Answer from the drawing. Dimensions are ordinates in mm from the lowest x, y and z of the part. Round coordinates to 2 decimals unless told otherwise and drop trailing zeros. Loops run counter-clockwise (first coordinate to the right, second up) from the corner with the lowest first, then second, coordinate; pieces in that order, holes last. Notation, with made-up numbers: (29, -7.5) - (38, -7.5) arc R9 ccw to (38, 7.5) - close; hole circle Ø10 at (6, -17.5). An arc over 180 degrees is marked (long way). Write item = value, one per line. Start each with the question number.
1) Section A-A, the plane y = 34 is taken. Determine the outline of the cut face in (x, z).
2) Given pin 1 Ø1.8 at (y, z) = (14.5, 4) entering from -X; pin 2 Ø3 at (x, z) = (254, 3.5) entering from -Y; pin 3 Ø3 at (x, z) = (95.5, 4) entering from +Y, each flat-ended and moving along its own axis, determine where each tip first touches the part or whether it passes through.
3) Section D-D, the plane y = 12.5 is taken. Determine the outline of the cut face in (x, z), and give its area (3 significant figures).
4) Straight lines are drawn through the part: line 1 along X through (y, z) = (63, 2.25); line 2 along Y through (x, z) = (34.5, 1.9); line 3 along Y through (x, z) = (224, 4.7). For each, find the intervals that lie inside material, in ascending order.
5) Section C-C, the plane x = 209.5 is taken. Determine the outline of the cut face in (y, z), and give its area (3 significant figures).
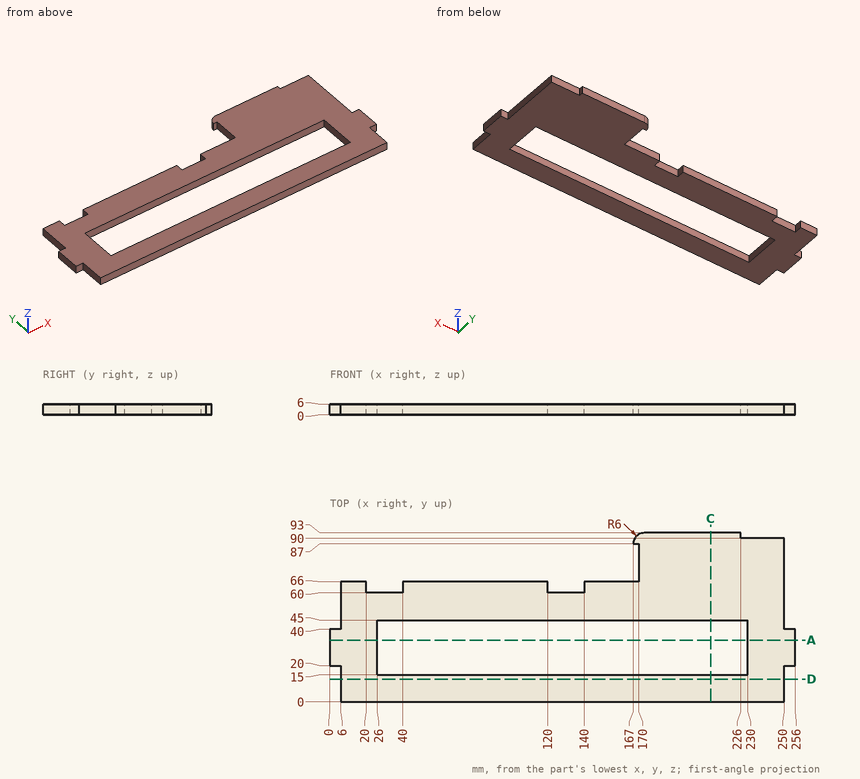
Geometry check:
q1.outline = (0, 0) - (26, 0) - (26, 6) - (0, 6) - close; (230, 0) - (256, 0) - (256, 6) - (230, 6) - close
q2.pin_1 = 6
q2.pin_2 = 20
q2.pin_3 = 66
q3.outline = (6, 0) - (250, 0) - (250, 6) - (6, 6) - close
q3.area = 1,460 mm2
q4.line_1 = 6 to 20, 40 to 120, 140 to 250
q4.line_2 = 0 to 15, 45 to 60
q4.line_3 = 0 to 15, 45 to 93
q5.outline = (0, 0) - (15, 0) - (15, 6) - (0, 6) - close; (45, 0) - (93, 0) - (93, 6) - (45, 6) - close
q5.area = 378 mm2
